from build123d import *

# Parameters (mm, degrees)
SKETCH1_R           = 7.5
BOSS_EXTRUDE1_DEPTH = 1
SKETCH4_R           = 4.5
BOSS_EXTRUDE2_DEPTH = 1
SKETCH5_R           = 1.6
CUT_EXTRUDE2_DEPTH  = 0.5
CHAMFER4_SIZE       = 2
CHAMFER4_SIZE_2     = 0.727940469
SKETCH6_R           = 1.5
CUT_EXTRUDE3_DEPTH  = 0.5


with BuildPart() as part:
    # Sketch1 → Boss-Extrude1 (new body)
    with BuildSketch(Plane.XY):
        Circle(SKETCH1_R)
    extrude(amount=BOSS_EXTRUDE1_DEPTH)

    # Sketch4 → Boss-Extrude2 (add)
    with BuildSketch(Plane.XY.offset(1)):
        Circle(SKETCH4_R)
    extrude(amount=BOSS_EXTRUDE2_DEPTH)

    # Sketch5 → Cut-Extrude2 (cut)
    with BuildSketch(Plane.XY.offset(2)):
        Circle(SKETCH5_R)
    extrude(amount=-CUT_EXTRUDE2_DEPTH, mode=Mode.SUBTRACT)

    # Chamfer4
    # the kernel refuses this chamfer: 2, 0.727940469 mm, written as the material it takes off along each edge
    with BuildSketch(Plane(origin=(0, 0, 2), x_dir=(1, 0, 0), z_dir=(0, -1, 0))) as chamfer4_piece_1_section:
        Polygon((4.5, -CHAMFER4_SIZE), (4.5 - CHAMFER4_SIZE_2, 0), (4.5, 0), align=None)
    chamfer4_piece_1 = revolve(axis=Axis((0, 0, 2), (0, 0, 1)), mode=Mode.PRIVATE)
    chamfer4_piece_1 = split(chamfer4_piece_1, bisect_by=Plane(origin=(-3.964304639, 0, 1), z_dir=(0, 0, 1)), keep=Keep.TOP, mode=Mode.PRIVATE)
    add(chamfer4_piece_1, mode=Mode.SUBTRACT)

    # Sketch6 → Cut-Extrude3 (cut)
    with BuildSketch(Plane(origin=(0, 0, 0), x_dir=(-1, 0, 0), z_dir=(0, 0, -1))):
        Circle(SKETCH6_R)
        with Locations((-4, 0)):
            Circle(SKETCH6_R)
        with Locations((0, 4)):
            Circle(SKETCH6_R)
        with Locations((4, 0)):
            Circle(SKETCH6_R)
        with Locations((0, -4)):
            Circle(SKETCH6_R)
    extrude(amount=-CUT_EXTRUDE3_DEPTH, mode=Mode.SUBTRACT)


solid = part.part
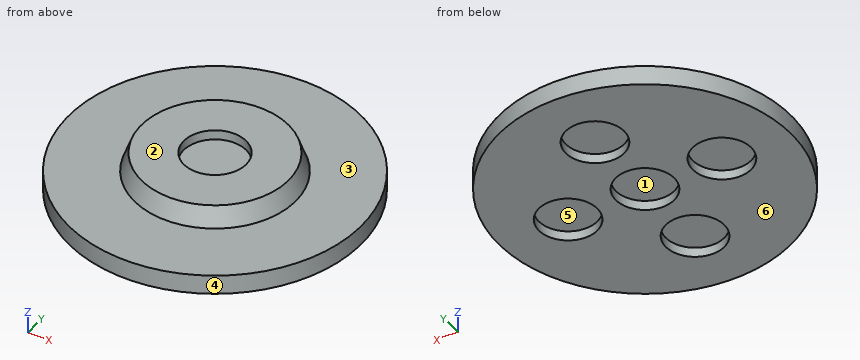
Can you work these out from the model? Positions are in its coordinate system, mm. Face numbers are marked on the shaded views. A direction names the side the tool comes from. Give positions to 0.01 mm unless a question says otherwise; leave off trailing zeros. Write each loop counter-clockwise with the first axis right and the second up, starting at its lowest first coordinate (ties: lowest second). Pieces come first, ordered by that corner, then holes. Notation, with made-up numbers: M -26.5,5.25 L 5.5,5.25 A28 cw 5.5,26.25 Z; hole C 75,-27.75 d3. An arc over 180 degrees is marked long. Answer in a Markdown table with one row per item. Add a question column.
Item 1: Please list where these lines run through material, in increasing order: L1, parallel to Y at x = 0, z = 0.3; L2, parallel to Z at x = 1.25, y = -0.75; L3, parallel to X at y = -1, z = 0.3.
Item 2: Imagine slicing it at A-A, the plane x = 0. Write out the boundary of the cut face in (y, z), plus the area to 3 significant figures.
Item 3: Imagine slicing it at C-C, the plane y = -5. Write out the boundary of the cut face in (x, z).
Item 4: For pin 1 Ø1.5 at (x, y) = (-4, 0.5) entering from -Z; pin 2 Ø3.5 at (x, y) = (0, -4) entering from -Z, each with a flat end and sliding along its axis, tell me the tip position at first contact or that it passes through.
Item 5: On a 3-axis mill with a long thin cutter (end or side, diameter ignored), from which of +Z, -Z, +X, -X, +Y, -Y can I reach the whole of each face in a straight line? I mean the marked faces 1, 2 and 3. Say none if no direction works.
Item 6: Imagine slicing it at D-D, the plane z = 1.3. Write out the boundary of the cut face in (x, y).
Item 7: We'd pull the mould along Y, two halves only. Please class the marked faces 4, 5 and 6: released by +Y, released by -Y, zero draft, split by the parting line, or undercut.
Evaluation:
| question | item | result |
|---|---|---|
| 1 | L1 | y = -7.5 to -5.5, -2.5 to -1.5, 1.5 to 2.5, 5.5 to 7.5 |
| 1 | L2 | z = 0.5 to 1.5 |
| 1 | L3 | x = -7.43 to -5.12, -2.88 to -1.12, 1.12 to 2.88, 5.12 to 7.43 |
| 2 | outline | M -7.5,0 L -5.5,0 L -5.5,0.5 L -2.5,0.5 L -2.5,0 L -1.5,0 L -1.5,0.5 L 1.5,0.5 L 1.5,0 L 2.5,0 L 2.5,0.5 L 5.5,0.5 L 5.5,0 L 7.5,0 L 7.5,1 L 4.14,1 L 3.77,2 L 1.6,2 L 1.6,1.5 L -1.6,1.5 L -1.6,2 L -3.77,2 L -4.14,1 L -7.5,1 Z |
| 2 | area | 16.8 mm² |
| 3 | outline | M -5.59,0 L -1.12,0 L -1.12,0.5 L 1.12,0.5 L 1.12,0 L 5.59,0 L 5.59,1 L -5.59,1 Z |
| 4 | pin 1 | stops at z = 0.5 |
| 4 | pin 2 | stops at z = 0 |
| 5 | face 1 | -Z |
| 5 | face 2 | +Z, +X, -X, +Y, -Y |
| 5 | face 3 | +Z |
| 6 | outline | C 0,0 d8.05 |
| 7 | face 4 | split by the parting line |
| 7 | face 5 | undercut |
| 7 | face 6 | zero draft |
